Could you check a few things on this drawing? It's one solid part, dimensions in mm from its lowest x, y, z. A direction names the side the tool comes from. Round coordinates to 2 decimals unless told otherwise and drop trailing zeros. Write each loop counter-clockwise with the first axis right and the second up, starting at its lowest first coordinate (ties: lowest second). Pieces come first, ordered by that corner, then holes. Notation, with made-up numbers: (56.5, 1.5) - (110.5, 1.5) arc R37 cw to (110.5, 39.5) - close; hole circle Ø3 at (76.25, 81.5). An arc over 180 degrees is marked (long way). Write item = value, one per line. Start each with the question number.
Item 1: Which directions (+Z, -Z, +X, -X, +Y, -Y) give clear straight access to the entire face, cutting with the end or side of a thin tool? Please do the marked faces 1, 2, 3 and 4.
Item 2: For P1, Ø0.7, axis at x = 4.5, z = 4, coming from the -Y side; P2, Ø1, axis at x = 4, y = 8.5, coming from the -Z side; P3, Ø1.5, axis at x = 6.5, y = 2.5, coming from the -Z side, each with a flat end and sliding along its axis, tell me the tip position at first contact or that it passes through.
Item 3: If we section it at B-B (x = 8): Please give me the cut outline in (y, z).
Item 4: If we section it at C-C (z = 4.3): Please give me the cut outline in (x, y), and give its area (3 significant figures).
Item 5: If we section it at A-A (y = 8): Please give me the cut outline in (x, z).
Item 6: Thinking about a two-plate mould opening in X: for the marked faces 5, 6 and 7, which applies, pulls with the +X half, pulls with the -X half, needs draft (parallel to the pull), parting line crosses it, or undercut?
Item 7: If I drill on line 1 along X through (y, z) = (1.6, 4.3); line 2 along Z through (x, y) = (2, 6); line 3 along X through (y, z) = (9, 1), over which ranges is the centre line in solid material (lowest first)? Write a range as [from, to].
Item 8: If we section it at D-D (y = 3.25): Please give me the cut outline in (x, z).
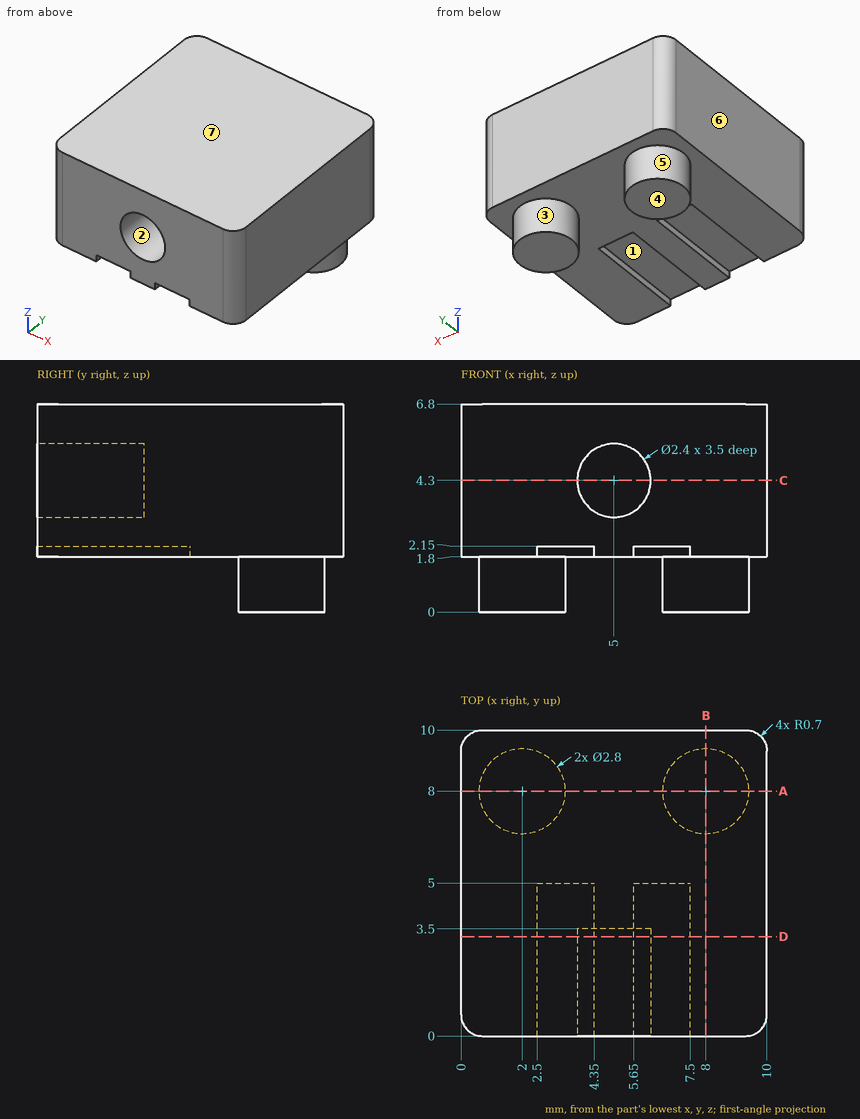
Reply:
q1.face_1 = -Z, -Y
q1.face_2 = -Y
q1.face_3 = -Z
q1.face_4 = -Z, +X, -X, +Y, -Y
q2.P1 = 3.5
q2.P2 = 1.8
q2.P3 = 2.15
q3.outline = (0, 1.8) - (6.6, 1.8) - (6.6, 0) - (9.4, 0) - (9.4, 1.8) - (10, 1.8) - (10, 6.8) - (0, 6.8) - close
q4.outline = (0, 0.7) arc R0.7 ccw to (0.7, 0) - (3.8, 0) - (3.8, 3.5) - (6.2, 3.5) - (6.2, 0) - (9.3, 0) arc R0.7 ccw to (10, 0.7) - (10, 9.3) arc R0.7 ccw to (9.3, 10) - (0.7, 10) arc R0.7 ccw to (0, 9.3) - close
q4.area = 91.2 mm2
q5.outline = (0, 1.8) - (0.6, 1.8) - (0.6, 0) - (3.4, 0) - (3.4, 1.8) - (6.6, 1.8) - (6.6, 0) - (9.4, 0) - (9.4, 1.8) - (10, 1.8) - (10, 6.8) - (0, 6.8) - close
q6.face_5 = undercut
q6.face_6 = pulls with the -X half
q6.face_7 = needs draft
q7.line_1 = [0, 3.8], [6.2, 10]
q7.line_2 = [1.8, 6.8]
q7.line_3 = [1.02, 2.98], [7.02, 8.98]
q8.outline = (0, 1.8) - (2.5, 1.8) - (2.5, 2.15) - (4.35, 2.15) - (4.35, 1.8) - (5.65, 1.8) - (5.65, 2.15) - (7.5, 2.15) - (7.5, 1.8) - (10, 1.8) - (10, 6.8) - (0, 6.8) - close; hole circle Ø2.4 at (5, 4.3)
